from build123d import *

# Parameters (mm, degrees)
SKETCH1_R                       = 3.175
BOSS_EXTRUDE1_DEPTH             = 12.7
SKETCH2_R                       = 7.9375
CUT_EXTRUDE1_DEPTH              = 6.35
F_1_4_0_25_DIAMETER_HOLE1_D     = 6.35
F_1_4_0_25_DIAMETER_HOLE1_DEPTH = 12.7
F_1_4_0_25_DIAMETER_HOLE1_TIP   = 1.907732465


with BuildPart() as part:
    # Sketch1 → Boss-Extrude1 (new body)
    # profile 1 of 2: a face of its own
    with BuildSketch(Plane(origin=(0, 0, 0), x_dir=(0, 0, -1), z_dir=(1, 0, 0))):
        with BuildLine():
            Line((-76.2, 38.1), (-76.2, 0))
            Line((-76.2, 0), (-41.275, 0))
            ThreePointArc((-41.275, 0), (-38.1, 3.175), (-34.925, 0))
            Line((-34.925, 0), (15.74272634, 0))
            ThreePointArc((15.74272634, 0), (18.16587039, 4.221897852), (21.89753158, 1.096077429))
            ThreePointArc((21.89753158, 1.096077429), (21.848352003, 0.539416238), (21.70233682, 0))
            Line((21.70233682, 0), (76.2, 0))
            Line((76.2, 0), (76.2, 38.1))
            Line((76.2, 38.1), (-76.2, 38.1))
        make_face()
    # profile 2 of 2: a face of its own
    with BuildSketch(Plane(origin=(0, 0, 0), x_dir=(0, 0, -1), z_dir=(1, 0, 0))):
        with BuildLine():
            Line((-41.275, 0), (-76.2, 0))
            Line((-76.2, 0), (-76.2, -38.1))
            Line((-76.2, -38.1), (76.2, -38.1))
            Line((76.2, -38.1), (76.2, 0))
            Line((76.2, 0), (21.70233682, 0))
            ThreePointArc((21.70233682, 0), (18.72253158, -2.078922571), (15.74272634, 0))
            Line((15.74272634, 0), (-34.925, 0))
            ThreePointArc((-34.925, 0), (-38.1, -3.175), (-41.275, 0))
        make_face()
        with Locations((-14.571224015, -7.860160654)):
            Circle(SKETCH1_R, mode=Mode.SUBTRACT)
        with Locations((51.408255992, -9.873506971)):
            Circle(SKETCH1_R, mode=Mode.SUBTRACT)
    extrude(amount=BOSS_EXTRUDE1_DEPTH)

    # Sketch2 → Cut-Extrude1 (cut)
    with BuildSketch(Plane.ZY):
        with Locations((38.1, 0)):
            Circle(SKETCH2_R)
        with Locations((14.571224015, -7.860160654)):
            Circle(SKETCH2_R)
        with Locations((-18.72253158, 1.096077429)):
            Circle(SKETCH2_R)
        with Locations((-51.408255992, -9.873506971)):
            Circle(SKETCH2_R)
    extrude(amount=-CUT_EXTRUDE1_DEPTH, mode=Mode.SUBTRACT)

    # 1_4 _0.25_ Diameter Hole1
    with Locations(Plane.XZ.offset(38.1)):
        with Locations((6.35, -63.5), (6.35, 0), (6.35, 57.15)):
            Hole(F_1_4_0_25_DIAMETER_HOLE1_D / 2, depth=F_1_4_0_25_DIAMETER_HOLE1_DEPTH)
            with Locations((0, 0, -(F_1_4_0_25_DIAMETER_HOLE1_DEPTH + F_1_4_0_25_DIAMETER_HOLE1_TIP / 2))):  # 118° drill point
                Cone(0, F_1_4_0_25_DIAMETER_HOLE1_D / 2, F_1_4_0_25_DIAMETER_HOLE1_TIP, mode=Mode.SUBTRACT)


solid = part.part
The listing builds one solid part. Answer for the finished solid, in the listing's coordinates (mm). A direction names the side the tool comes from. Give positions to 0.01 mm unless a question says otherwise; leave off trailing zeros. Order: outer loops, then holes, each group sorted by start corner. A loop starts at its lowest first (then second) coordinate and runs counter-clockwise, first axis right, second up. Notation, with made-up numbers: (77.25, 70) - (113.25, 70) arc R16 ccw to (113.25, 90) - close; hole circle Ø2 at (64.5, -25.5). An arc over 180 degrees is marked (long way). One line per item, written item: value. Start each with the question number.
1) Given pin 1 Ø8 at (y, z) = (-8, -48) entering from -X, flat-ended and moving along its own axis, determine where the tip first touches the part or whether it passes through.
2) Find the intervals of material crossed by L1, parallel to X at y = -35, z = -63.5 (3 decimals); L2, parallel to Y at x = 7.75, z = -51; L3, parallel to Z at x = 5.25, y = -34, in increasing order.
3) A cutting plane is placed at D-D on z = 13.5. Give the vertices of the cut face in (x, y), then the cut area to 3 significant figures.
4) A cutting plane is placed at B-B on y = -27.5. Give the vertices of the cut face in (x, z) (3 decimals), then the cut area to 3 significant figures.
5) A tool of negligible diameter and unlimited length cuts with its end or side. For faces 1 (the face through (7.04, -31.66, 54.05)), 2 (the face through (9.48, 0.14, 34.93)), 3 (the face through (3.131, -9.525, -59.338)), from which of +Z, -Z, +X, -X, +Y, -Y can it reach the whole face along a straight path? Write none if from no direction.
6) A cutting plane is placed at C-C on z = -56.5. Give the vertices of the cut face in (x, y).
7) The mould has two halves that part along Z. Classify faces 4 (the face through (12.7, 1, 1)), 5 (the face through (6, -1, -76.2)), 6 (the face through (9.48, -11.09, -54.34)): released by +Z, released by -Z, zero draft, split by the parting line, or undercut.
Answer sheet:
1. pin 1: stops at x = 6.35
2. L1: x = 0 to 3.175, 9.525 to 12.7
2. L2: y = -38.1 to -13.02, -6.72 to 38.1
2. L3: z = -76.2 to -66.48, -60.52 to -2.98, 2.98 to 54.17, 60.13 to 76.2
3. outline: (0, -38.1) - (12.7, -38.1) - (12.7, -10.85) - (6.35, -10.85) - (6.35, -15.73) - (0, -15.73) - close; (0, 0) - (6.35, 0) - (6.35, -4.87) - (12.7, -4.87) - (12.7, 38.1) - (0, 38.1) - close
3. area: 830 mm2
4. outline: (0, -76.2) - (12.7, -76.2) - (12.7, 76.2) - (0, 76.2) - close; hole circle Ø6.35 at (6.35, -63.5); hole circle Ø6.35 at (6.35, 0); hole circle Ø6.35 at (6.35, 57.15)
4. area: 1,840 mm2
5. face 1: -Y
5. face 2: +X, -X
5. face 3: -X
6. outline: (0, -38.1) - (12.7, -38.1) - (12.7, 38.1) - (0, 38.1) - (0, -3.78) - (6.35, -3.78) - (6.35, -15.96) - (0, -15.96) - close
7. face 4: zero draft
7. face 5: released by -Z
7. face 6: undercut
